Autodesk Inventor part; units mm, degrees
ref_plane "YZ Plane" through (0, 0, 0) normal (1, 0, 0) x (0, 1, 0)
ref_plane "XZ Plane" through (0, 0, 0) normal (0, 1, 0) x (-1, 0, 0)
ref_plane "XY Plane" through (0, 0, 0) normal (0, 0, 1) x (1, 0, 0)
sketch "スケッチ1" plane through (0, 0, 0) normal (0, 0, 1) x (1, 0, 0)
  circle A0 centre (0, 0) radius 3
  dimension "d0" = 6
extrude "押し出し1" add sketch "スケッチ1" along normal blind 20
chamfer "面取り1" distance 1.2 angle 15 2 edges at (-3, 0, 20) (-3, 0, 0) measured on face at (2.9612, -0.4812, 13.3333)
sketch "スケッチ2" plane through (0, 0, 0) normal (0, 0, -1) x (-1, 0, 0)
  circle A0 centre (0, 0) radius 2
  dimension "d6" = 4
extrude "押し出し2" cut sketch "スケッチ2" against normal blind 8
properties part number "平行ピンΦ6.20 片雌ネジ" material "鋼、高強度、低合金"
Input: part model. Units: mm. Frame: model coordinates. A direction names the side the tool comes from. Give positions to 0.01 mm unless a question says otherwise; leave off trailing zeros. Order: outer loops, then holes, each group sorted by start corner. A loop starts at its lowest first (then second) coordinate and runs counter-clockwise, first axis right, second up.
1. Line query: probe 1 along Y at (x, z) = (0, 6); probe 2 along Z at (x, y) = (-0.55, -0.3); probe 3 along Y at (x, z) = (0.6, 6.25). Output: solid intervals per line, ascending.
Computed:
probe 1: y = -3 to -2, 2 to 3
probe 2: z = 8 to 20
probe 3: y = -2.94 to -1.91, 1.91 to 2.94
2. Cut plane C-C (z = 5.75). Return loops of the section in (x, y).
Computed:
outline: circle Ø6 at (0, 0); hole circle Ø4 at (0, 0)
3. Set-up query: faces 1 (the face through (0, 0, 8)), 2 (the face through (0, 0, 20)). Return all of +Z, -Z, +X, -X, +Y, -Y with unobstructed straight access to the full face (end or side cutting, diameter ignored); none if empty.
Computed:
face 1: -Z
face 2: +Z, +X, -X, +Y, -Y
4. Cut plane A-A (x = 0). Return loops of the section in (y, z), and give its area (3 significant figures).
Computed:
outline: (-3, 1.2) - (-2.68, 0) - (-2, 0) - (-2, 8) - (2, 8) - (2, 0) - (2.68, 0) - (3, 1.2) - (3, 18.8) - (2.68, 20) - (-2.68, 20) - (-3, 18.8) - close
area: 87.2 mm2
5. Pin query (flat end, axial travel): pin 1 Ø2 at (x, y) = (-0.5, 0.5) entering from -Z; pin 2 Ø1 at (y, z) = (-2, 5.5) entering from +X; pin 3 Ø1.5 at (y, z) = (1, 8.5) entering from -X. Return the tip coordinate at first contact, or that it passes through.
Computed:
pin 1: stops at z = 8
pin 2: stops at x = 2.6
pin 3: stops at x = -2.99
6. Cut plane D-D (z = 16.75). Return loops of the section in (x, y), and give its area (3 significant figures).
Computed:
outline: circle Ø6 at (0, 0)
area: 28.3 mm2
7. Draft query along X for faces 3 (the face through (0, -2, 4)), 4 (the face through (-1, -2, 0)), 5 (the face through (-3, 0, 10)). Return one class per face: released by +X, released by -X, zero draft, split by the parting line, or undercut.
Computed:
face 3: undercut
face 4: zero draft
face 5: split by the parting line
